from build123d import *

# Parameters (mm, degrees)
ESQUISSE5_W             = 61
ESQUISSE5_H             = 27
BOSS_EXTRU_2_DEPTH      = 16.5
ENL_V_MAT_EXTRU_2_DEPTH = 16.5
ESQUISSE7_W             = 10
ESQUISSE7_H             = 27
BOSS_EXTRU_3_DEPTH      = 32
ESQUISSE8_R             = 2
ENL_V_MAT_EXTRU_3_DEPTH = 40
ESQUISSE9_R             = 3.75
ENL_V_MAT_EXTRU_4_DEPTH = 4
CHANFREIN1_SIZE         = 2
CHANFREIN2_SIZE         = 3
ESQUISSE10_W            = 6
ESQUISSE10_H            = 6
ENL_V_MAT_EXTRU_5_DEPTH = 36
ESQUISSE11_R            = 2.25
ENL_V_MAT_EXTRU_6_DEPTH = 8
ESQUISSE12_R            = 1.5
ENL_V_MAT_EXTRU_7_DEPTH = 8
CHANFREIN3_SIZE         = 3


with BuildPart() as part:
    # Esquisse5 → Boss.-Extru.2 (new body)
    with BuildSketch(Plane.XY):
        Rectangle(ESQUISSE5_W, ESQUISSE5_H)
    extrude(amount=BOSS_EXTRU_2_DEPTH)

    # Esquisse6 → Enlèv. mat.-Extru.2 (cut)
    with BuildSketch(Plane.XY.offset(16.5)):
        with BuildLine():
            Line((-4, 38.524390244), (4, 38.524390244))
            Line((4, 38.524390244), (4, 3.5))
            ThreePointArc((4, 3.5), (0, -0.5), (-4, 3.5))
            Line((-4, 3.5), (-4, 38.524390244))
        make_face()
    extrude(amount=-ENL_V_MAT_EXTRU_2_DEPTH, mode=Mode.SUBTRACT)

    # Esquisse7 → Boss.-Extru.3 (add)
    with BuildSketch(Plane(origin=(0, 0, 0), x_dir=(-1, 0, 0), z_dir=(0, 0, -1))):
        with Locations((-35.5, 0)):
            Rectangle(ESQUISSE7_W, ESQUISSE7_H)
        with Locations((35.5, 0)):
            Rectangle(ESQUISSE7_W, ESQUISSE7_H)
    extrude(amount=-BOSS_EXTRU_3_DEPTH)

    # Esquisse8 → Enlèv. mat.-Extru.3 (cut)
    with BuildSketch(Plane.XY.offset(32)):
        with Locations((-35.5, 0)):
            Circle(ESQUISSE8_R)
        with Locations((35.5, 0)):
            Circle(ESQUISSE8_R)
    extrude(amount=-ENL_V_MAT_EXTRU_3_DEPTH, mode=Mode.SUBTRACT)

    # Esquisse9 → Enlèv. mat.-Extru.4 (cut)
    with BuildSketch(Plane(origin=(0, 0, 0), x_dir=(-1, 0, 0), z_dir=(0, 0, -1))):
        with Locations((-35.5, 0)):
            Circle(ESQUISSE9_R)
        with Locations((35.5, 0)):
            Circle(ESQUISSE9_R)
    extrude(amount=-ENL_V_MAT_EXTRU_4_DEPTH, mode=Mode.SUBTRACT)

    # Chanfrein1
    chanfrein1_edges = [part.edges().sort_by_distance(p)[0] for p in [
        (-4, 13.5, 8.25),
        (4, 13.5, 8.25),
    ]]
    chamfer(chanfrein1_edges, length=CHANFREIN1_SIZE)

    # Chanfrein2
    chanfrein2_edges = [part.edges().sort_by_distance(p)[0] for p in [
        (30.5, 13.5, 24.25),
        (-30.5, 13.5, 24.25),
    ]]
    chamfer(chanfrein2_edges, length=CHANFREIN2_SIZE)

    # Esquisse10 → Enlèv. mat.-Extru.5 (cut)
    with BuildSketch(Plane(origin=(0, 13.5, 0), x_dir=(1, 0, 0), z_dir=(0, 1, 0))):
        with Locations((24, -13.5)):
            Rectangle(ESQUISSE10_W, ESQUISSE10_H)
    extrude(amount=-ENL_V_MAT_EXTRU_5_DEPTH, mode=Mode.SUBTRACT)

    # Esquisse11 → Enlèv. mat.-Extru.6 (cut)
    with BuildSketch(Plane.XY.offset(10.5)):
        with Locations((24, 8.5)):
            Circle(ESQUISSE11_R)
        with Locations((24, -8.5)):
            Circle(ESQUISSE11_R)
    extrude(amount=-ENL_V_MAT_EXTRU_6_DEPTH, mode=Mode.SUBTRACT)

    # Esquisse12 → Enlèv. mat.-Extru.7 (cut)
    with BuildSketch(Plane.XY.offset(2.5)):
        with Locations((24, 8.5)):
            Circle(ESQUISSE12_R)
        with Locations((24, -8.5)):
            Circle(ESQUISSE12_R)
    extrude(amount=-ENL_V_MAT_EXTRU_7_DEPTH, mode=Mode.SUBTRACT)

    # Chanfrein3
    chanfrein3_edges = [part.edges().sort_by_distance(p)[0] for p in [
        (30.25, 13.5, 16.5),
        (13.5, 13.5, 16.5),
        (-19.75, 13.5, 16.5),
    ]]
    chamfer(chanfrein3_edges, length=CHANFREIN3_SIZE)


solid = part.part
CAD build for the part. Positions are in the model's coordinates, mm. A direction names the side the tool comes from. Coordinates: 2 decimals unless noted, no trailing zeros. Write each loop counter-clockwise with the first axis right and the second up, starting at its lowest first coordinate (ties: lowest second). Pieces come first, ordered by that corner, then holes. Notation, with made-up numbers: M -23.5,58 L 17.5,58 A18 cw 17.5,75 Z; hole C 81,24 d2. An arc over 180 degrees is marked long. Return JSON: item names as keys, results as strings.
Item 1: Probe line 1 (X direction, y = -8.5, z = 24); line 2 (Y direction, x = 24, z = 4); line 3 (X direction, y = -6.75, z = 14). List the from-to ranges inside material, lowest first. Write a range as from..to.
Findings below:
{"line 1": "x = -40.5..-30.5, 30.5..40.5", "line 2": "y = -13.5..-10.75, -6.25..6.25, 10.75..13.5", "line 3": "x = -40.5..21, 27..40.5"}
Item 2: Slice it at C-C, the plane x = 24. Write the cut outline in (y, z).
Findings below:
{"outline": "M -13.5,0 L -10,0 L -10,2.5 L -10.75,2.5 L -10.75,10.5 L -13.5,10.5 Z; M -7,0 L 7,0 L 7,2.5 L 6.25,2.5 L 6.25,10.5 L -6.25,10.5 L -6.25,2.5 L -7,2.5 Z; M 10,0 L 13.5,0 L 13.5,10.5 L 10.75,10.5 L 10.75,2.5 L 10,2.5 Z"}
Item 3: Which spindle directions (+Z, -Z, +X, -X, +Y, -Y) get a long thin tool onto all of the face, cutting with end or side? Do faces 1 (the flat face through (12, 12, 15)), 2 (the flat face through (-4, 7, 8)), 3 (the flat face through (30.5, -2, 24)). Say none if no direction does.
Findings below:
{"face 1": "+Z, +Y", "face 2": "+Z, -Z, +Y", "face 3": "+Z, +Y, -Y"}
Item 4: Slice it at D-D, the plane y = -8.5. Write the cut outline in (x, z).
Findings below:
{"outline": "M -40.5,0 L 22.5,0 L 22.5,2.5 L 21.75,2.5 L 21.75,10.5 L 21,10.5 L 21,16.5 L -30.5,16.5 L -30.5,32 L -40.5,32 Z; M 25.5,0 L 40.5,0 L 40.5,32 L 30.5,32 L 30.5,16.5 L 27,16.5 L 27,10.5 L 26.25,10.5 L 26.25,2.5 L 25.5,2.5 Z"}
Item 5: Slice it at B-B, the plane y = 8.5. Write the cut outline in (x, z).
Findings below:
{"outline": "M -40.5,0 L -4,0 L -4,16.5 L -30.5,16.5 L -30.5,32 L -40.5,32 Z; M 4,0 L 22.5,0 L 22.5,2.5 L 21.75,2.5 L 21.75,10.5 L 21,10.5 L 21,16.5 L 4,16.5 Z; M 25.5,0 L 40.5,0 L 40.5,32 L 30.5,32 L 30.5,16.5 L 27,16.5 L 27,10.5 L 26.25,10.5 L 26.25,2.5 L 25.5,2.5 Z"}
Item 6: Slice it at A-A, the plane z = 23. Write the cut outline in (x, y), and give its area (3 significant figures).
Findings below:
{"outline": "M -40.5,-13.5 L -30.5,-13.5 L -30.5,10.5 L -33.5,13.5 L -40.5,13.5 Z; M 30.5,-13.5 L 40.5,-13.5 L 40.5,13.5 L 33.5,13.5 L 30.5,10.5 Z; hole C -35.5,0 d4; hole C 35.5,0 d4", "area": "506 mm2"}
Item 7: Two-plate mould, pull along Y, no slides. Class faces 4 (the cylindrical face through (26.146, -7.824, 6.556)), 5 (the flat face through (29, -1, 16.5)), 6 (the flat face through (-32, 12, 23)): +Y half, -Y half, draft (parallel to the pull), parting line (faces both ways), or undercut.
Findings below:
{"face 4": "undercut", "face 5": "draft", "face 6": "+Y half"}
Item 8: Drop flat-ended pins along their axis: pin 1 Ø1.8 at (x, y) = (25.5, 6.5) entering from +Z; pin 2 Ø8 at (x, y) = (14.5, 8.5) entering from +Z; pin 3 Ø3.5 at (x, y) = (24, 8.5) entering from +Z. Give the stop position or say it passes through.
Findings below:
{"pin 1": "stops at z = 10.5", "pin 2": "stops at z = 16.5", "pin 3": "stops at z = 2.5"}
